```python
from build123d import *

# Parameters (mm, degrees)
F0_W     = 40
F0_H     = 35
F0_R     = 3
F1_DEPTH = 8
F2_DEPTH = 2
F3_W     = 40
F3_H     = 27
F4_DEPTH = 3
F5_R     = 20
F6_R     = 19.99999
F8_DEPTH = 2.001
F9_DEPTH = 2.001


# Not quite as in the source:
# - a fillet or chamfer is up to 0.001 mm smaller than in the source, because OpenCascade refuses the exact size


with BuildPart() as f1:
    # F0 (on Top) → F1 (new body)
    with BuildSketch(Plane.XY):
        Rectangle(F0_W, F0_H)
        with Locations((0, 2.5)):
            Circle(F0_R, mode=Mode.SUBTRACT)
    extrude(amount=F1_DEPTH)

    # F0 (on Top) → F2 (join)
    with BuildSketch(Plane.XY):
        with Locations((0, 2.5)):
            Circle(F0_R)
    extrude(amount=F2_DEPTH)

    # F3 (on face) → F4 (join)
    with BuildSketch(Plane.XZ.offset(17.5)):
        with Locations((0, 21.5)):
            Rectangle(F3_W, F3_H)
    extrude(amount=-F4_DEPTH)

    # F5
    f5_edges = [f1.edges().sort_by_distance(p)[0] for p in [
        (-20, 17.5, 4),
    ]]
    fillet(f5_edges, radius=F5_R)

    # F6 (radius 20 in the source; OpenCascade refuses exactly that, so slightly less here)
    f6_edges = [f1.edges().sort_by_distance(p)[0] for p in [
        (20, 17.5, 4),
    ]]
    fillet(f6_edges, radius=F6_R)

    # F7: F1 across face


with BuildPart() as f1_1:
    add(f1.part)
    add(f1.part.mirror(Plane(origin=(0, -16, 35), x_dir=(1, 0, 0), z_dir=(0, 0, 1))))

    # F8 (cut, through all): a face of the model
    f8_faces = [f1_1.faces().sort_by_distance(p)[0] for p in [
        (0, 2.5, 2),
    ]]
    extrude(f8_faces, amount=-F8_DEPTH, mode=Mode.SUBTRACT)

    # F9 (cut, through all): a face of the model
    f9_faces = [f1_1.faces().sort_by_distance(p)[0] for p in [
        (0, 2.5, 68),
    ]]
    extrude(f9_faces, amount=-F9_DEPTH, mode=Mode.SUBTRACT)


solid = f1_1.part
```
The model under review builds one solid part; all positions refer to its coordinate system, in mm. A direction names the side the tool comes from. Coordinates: 2 decimals unless noted, no trailing zeros. Order: outer loops, then holes, each group sorted by start corner. A loop starts at its lowest first (then second) coordinate and runs counter-clockwise, first axis right, second up. Notation, with made-up numbers: (20, 81) -> (62, 81) arc R23 cw to (62, 95) -> close; hole circle Ø11 at (40, 15.5). An arc over 180 degrees is marked (long way). Answer in a Markdown table with one row per item. Add a question column.
Item 1: Mouldability with a two-part tool opening along Z and no side actions: class faces 1 (the flat face through (0, -4, 0)), 2 (the cylindrical face through (-14.297, 11.486, 4.056)), 3 (the flat face through (0, -2, 8)), 4 (the flat face through (0, -14.5, 35)) as +Z half, -Z half, draft (parallel to the pull), parting line (faces both ways), or undercut.
Item 2: Machinability: for faces 5 (the cylindrical face through (-14.297, 11.486, 65.944)), 6 (the flat face through (0, -2, 62)), which of the approach directions +Z, -Z, +X, -X, +Y, -Y give a long, thin tool a straight path to every point of the face, cutting with its end or side? Answer none if there is none.
Item 3: To check wall thickness, follow probe 1 along Z at (x, y) = (3, 4.5); probe 2 along Y at (x, z) = (0, 0.8); probe 3 along Y at (x, z) = (5.5, 54). State the ranges of each line that lie inside material, in increasing order.
Item 4: Clearance check with a flat-ended pin moving along its axis: pin 1 (12 mm diameter, centred on x = 2.5, z = 25, fed in from +Y). State where the tip first meets the part, or that it passes through.
Item 5: We need section D-D on x = -12. Write out the cut boundary in (y, z).
Item 6: We need section C-C on y = 2.5. Write out the cut boundary in (x, z), plus the area to 3 significant figures.
Item 7: We need section A-A on y = -8. Write out the cut boundary in (x, z), plus the area to 3 significant figures.
Final values:
| question | item | result |
|---|---|---|
| 1 | face 1 | -Z half |
| 1 | face 2 | draft |
| 1 | face 3 | undercut |
| 1 | face 4 | undercut |
| 2 | face 5 | +Z, -Z, -X, +Y |
| 2 | face 6 | +X, -X, +Y |
| 3 | probe 1 | z = 0 to 8, 62 to 70 |
| 3 | probe 2 | y = -17.5 to -0.5, 5.5 to 17.5 |
| 3 | probe 3 | y = -17.5 to -14.5 |
| 4 | pin 1 | stops at y = -14.5 |
| 5 | outline | (-17.5, 0) -> (13.5, 0) -> (13.5, 8) -> (-14.5, 8) -> (-14.5, 62) -> (13.5, 62) -> (13.5, 70) -> (-17.5, 70) -> close |
| 6 | outline | (-19.36, 0) -> (-3, 0) -> (-3, 8) -> (-19.36, 8) -> close; (-19.36, 62) -> (-3, 62) -> (-3, 70) -> (-19.36, 70) -> close; (3, 0) -> (19.36, 0) -> (19.36, 8) -> (3, 8) -> close; (3, 62) -> (19.36, 62) -> (19.36, 70) -> (3, 70) -> close |
| 6 | area | 524 mm2 |
| 7 | outline | (-20, 0) -> (20, 0) -> (20, 8) -> (-20, 8) -> close; (-20, 62) -> (20, 62) -> (20, 70) -> (-20, 70) -> close |
| 7 | area | 640 mm2 |
